from build123d import *

# Parameters (mm, degrees)
SKETCH1_R           = 1.1811
RODEND_DEPTH        = 7.62
SKETCH4_R           = 1.1811
REVOLVE1_ANGLE      = 90
SKETCH5_R           = 1.1811
BOSS_EXTRUDE1_DEPTH = 152.4
SKETCH6_R           = 1.1811
REVOLVE2_ANGLE      = 15
SKETCH7_R           = 1.1811
BOSS_EXTRUDE2_DEPTH = 5.08


with BuildPart() as part:
    # Sketch1 → RodEnd (new body)
    with BuildSketch(Plane.XY):
        Circle(SKETCH1_R)
    extrude(amount=-RODEND_DEPTH)

    # Sketch4 → Revolve1 (revolve)
    with BuildSketch(Plane(origin=(0, 0, -7.62), x_dir=(-1, 0, 0), z_dir=(0, 0, -1))):
        with Locations(Location((0, 0, 0), (0, 0, 180))):
            Circle(SKETCH4_R)
    revolve(axis=Axis((-6.35, 0, -7.62), (0, 1, 0)), revolution_arc=REVOLVE1_ANGLE)

    # Sketch5 → Boss-Extrude1 (add)
    with BuildSketch(Plane.ZY.offset(6.35)):
        with Locations(Location((-13.97, 0, 0), (0, 0, 180))):
            Circle(SKETCH5_R)
    extrude(amount=BOSS_EXTRUDE1_DEPTH)

    # Sketch6 → Revolve2 (revolve)
    with BuildSketch(Plane.XY):
        Circle(SKETCH6_R)
    revolve(axis=Axis((0, -1.27, 0), (1, 0, 0)), revolution_arc=REVOLVE2_ANGLE)

    # Sketch7 → Boss-Extrude2 (add)
    with BuildSketch(Plane(origin=(0, -0.085073869, 0.3175), x_dir=(-1, 0, 0), z_dir=(0, -0.25881904510252135, 0.9659258262890682))):
        with Locations(Location((0, -0.043274201, 0), (0, 0, 270))):
            Circle(SKETCH7_R)
    extrude(amount=BOSS_EXTRUDE2_DEPTH)


solid = part.part
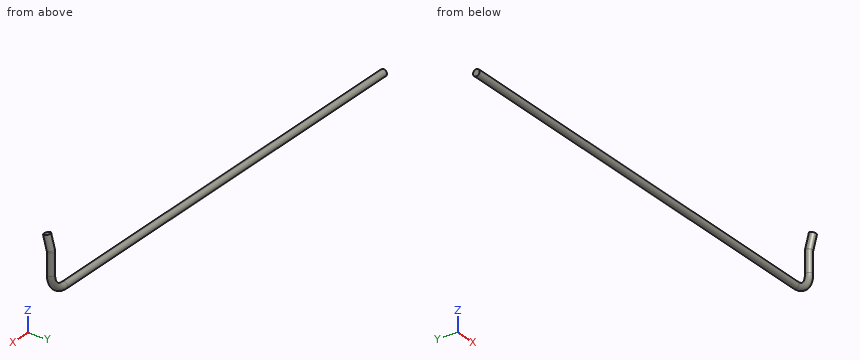
The listing builds one solid part. Answer for the finished solid, in the listing's coordinates (mm). Give positions to 0.01 mm unless a question says otherwise; leave off trailing zeros. Write each loop counter-clockwise with the first axis right and the second up, starting at its lowest first coordinate (ties: lowest second). Pieces come first, ordered by that corner, then holes.
1) Given P1, Ø2, axis at y = -2, z = -1, coming from the -X side, flat-ended and moving along its own axis, determine where the tip first touches the part or whether it passes through.
2) Find the intervals of material crossed by L1, parallel to X at y = 0.25, z = -6.75; L2, parallel to Z at x = -137.5, y = 0.1; L3, parallel to X at y = -1.6, z = 2.75, in increasing order.
3) Section B-B (x = -95) is taken. Write down the section's boundary in (y, z), and give its area (3 significant figures).
4) Section A-A (z = -5.75) is taken. Write down the section's boundary in (x, y).
Response:
1. P1: stops at x = -0.63
2. L1: x = -1.15 to 1.15
2. L2: z = -15.15 to -12.79
2. L3: x = -0.79 to 0.79
3. outline: circle Ø2.36 at (0, -13.97)
3. area: 4.38 mm2
4. outline: circle Ø2.36 at (0, 0)
